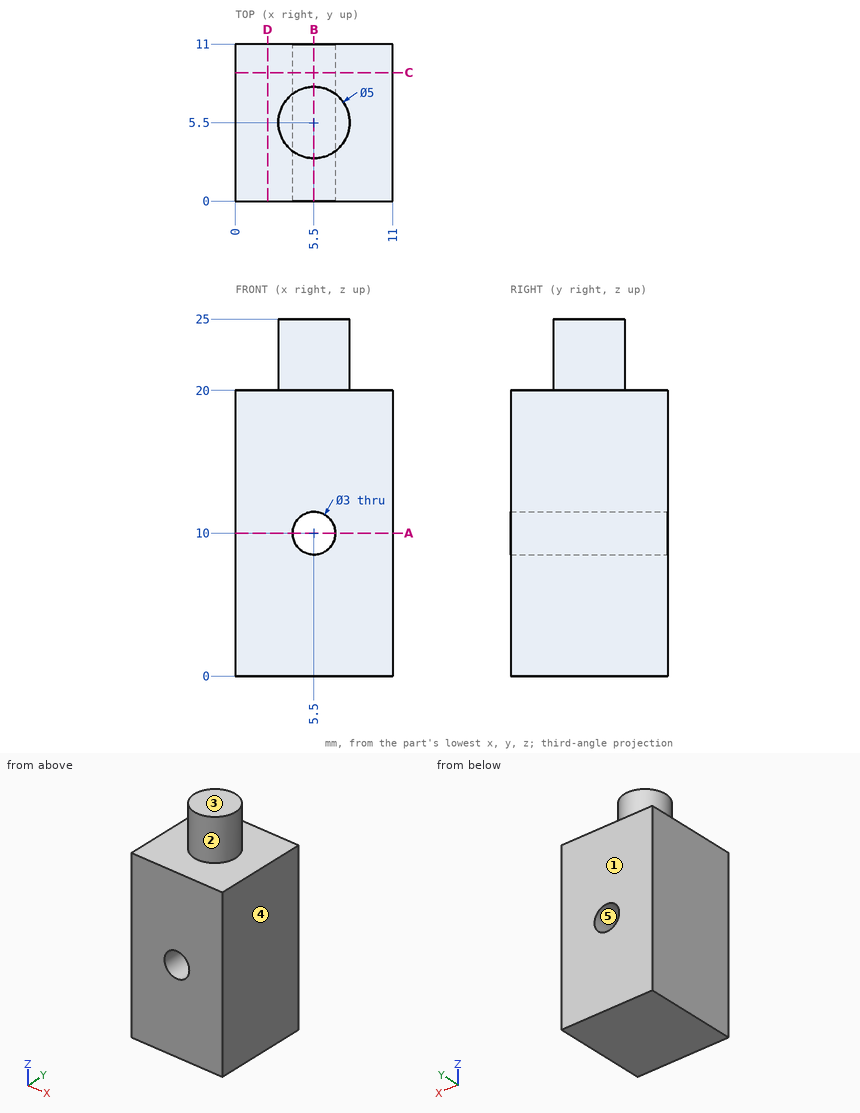
Input: dimensioned drawing with shaded views. Units: mm. Origin: part minimum x, y, z. A direction names the side the tool comes from. Give positions to 0.01 mm unless a question says otherwise; leave off trailing zeros. Write each loop counter-clockwise with the first axis right and the second up, starting at its lowest first coordinate (ties: lowest second). Pieces come first, ordered by that corner, then holes.
Q1. Section D-D, the plane x = 2.25. Output: boundary loops of the cut face in (y, z), plus the area to 3 significant figures.
Q2. Section A-A, the plane z = 10. Output: boundary loops of the cut face in (x, y).
Q3. Section C-C, the plane y = 9. Output: boundary loops of the cut face in (x, z), plus the area to 3 significant figures.
Q4. Pull-direction query (X, two-part tool) for the marked faces 3, 4 and 5; classes: pulls with the +X half, pulls with the -X half, needs draft (parallel to the pull), parting line crosses it, or undercut.
Q5. Section B-B, the plane x = 5.5. Output: boundary loops of the cut face in (y, z).
Q6. Set-up query: the marked faces 1 and 2. Return all of +Z, -Z, +X, -X, +Y, -Y with unobstructed straight access to the full face (end or side cutting, diameter ignored); none if empty.
Q7. Material intervals for probe 1 along X at (y, z) = (7, 10); probe 2 along Z at (x, y) = (5.5, 6.5); probe 3 along Z at (x, y) = (1.25, 1), sorted ascending.
Filled in:
1. outline: (0, 0) - (11, 0) - (11, 20) - (0, 20) - close
1. area: 220 mm2
2. outline: (0, 0) - (4, 0) - (4, 11) - (0, 11) - close; (7, 0) - (11, 0) - (11, 11) - (7, 11) - close
3. outline: (0, 0) - (11, 0) - (11, 20) - (0, 20) - close; hole circle Ø3 at (5.5, 10)
3. area: 213 mm2
4. face 3: needs draft
4. face 4: pulls with the +X half
4. face 5: undercut
5. outline: (0, 0) - (11, 0) - (11, 8.5) - (0, 8.5) - close; (0, 11.5) - (11, 11.5) - (11, 20) - (8, 20) - (8, 25) - (3, 25) - (3, 20) - (0, 20) - close
6. face 1: +Z, -Z, +X, -X, +Y
6. face 2: +Z
7. probe 1: x = 0 to 4, 7 to 11
7. probe 2: z = 0 to 8.5, 11.5 to 25
7. probe 3: z = 0 to 20
